Can you work these out from the model? Positions are in its coordinate system, mm. Face numbers are marked on the shaded views. A direction names the side the tool comes from. Round coordinates to 2 decimals unless told otherwise and drop trailing zeros. Loops run counter-clockwise (first coordinate to the right, second up) from the corner with the lowest first, then second, coordinate; pieces in that order, holes last.
(1) I want a section at A-A on x = 10.75. Write out the boundary of the cut face in (y, z), plus the area to 3 significant figures.
(2) I want a section at B-B on y = -11. Write out the boundary of the cut face in (x, z), plus the area to 3 significant figures.
(3) Will these pins go through, and if not, where does the flat tip stop? pin 1 Ø0.5 at (x, z) = (4, -18.5) entering from -Y; pin 2 Ø5.5 at (y, z) = (-0.5, -9) entering from -X.
(4) Which directions (+Z, -Z, +X, -X, +Y, -Y) give clear straight access to the entire face, cutting with the end or side of a thin tool? Please do the marked faces 5, 6, 7 and 8.
(5) Thinking about a two-plate mould opening in X: for the marked faces 1, 2, 3 and 4, which applies, released by +X, released by -X, zero draft, split by the parting line, or undercut?
(6) I want a section at C-C on y = -8.25. Write out the boundary of the cut face in (x, z) (3 decimals).
(7) If I drill on line 1 along Z through (x, y) = (19, -5.5); line 2 along Z through (x, y) = (24.5, 3); line 3 along Y through (x, z) = (25.25, -12) (3 decimals), over which ranges is the centre line in solid material (lowest first)?
from build123d import *

# Parameters (mm, degrees)
BLANKSKE_W           = 27
BLANKSKE_H           = 13.325
BLANK_DEPTH          = 29
TOOTHCUTSIM_DEPTH    = 42.803775248
TEETHCUTS_COUNT      = 8
TEETHCUTS_PITCH      = 3.926990813
CUT_EXTRUDE1_DEPTH   = 6.75
SKETCH3_R            = 5.25
CUT_EXTRUDE2_DEPTH   = 10.25
SKETCH4_R            = 4.5
CUT_EXTRUDE3_DEPTH   = 37.16013862
SKETCH5_R            = 2.5
CUT_EXTRUDE4_DEPTH   = 3.175
SKETCH6_R            = 1.75
CUT_EXTRUDE5_DEPTH   = 40.826953813
MIRROR1_COPY_1_DEPTH = 42.803775248
MIRROR1_COPY_2_DEPTH = 42.803775248
MIRROR1_COPY_3_DEPTH = 42.803775248
MIRROR1_COPY_4_DEPTH = 42.803775248
MIRROR1_COPY_5_DEPTH = 42.803775248
MIRROR1_COPY_6_DEPTH = 42.803775248
MIRROR1_COPY_7_DEPTH = 42.803775248
SKETCH9_W            = 18.526
SKETCH9_H            = 18.526
CUT_EXTRUDE6_DEPTH   = 3.175


with BuildPart() as part:
    # BlankSke → Blank (new body)
    with BuildSketch(Plane.XY):
        with Locations((13.5, 6.6625)):
            Rectangle(BLANKSKE_W, BLANKSKE_H)
    blank = extrude(amount=-BLANK_DEPTH)

    # TooCutSkeSim → ToothCutSim (cut, through all)
    with BuildSketch(Plane.XY):
        Polygon((0.548044212, 10.5125), (-0.548044212, 10.5125), (-1.58095534, 13.3504), (1.58095534, 13.3504), align=None)
    toothcutsim = extrude(amount=-TOOTHCUTSIM_DEPTH, mode=Mode.SUBTRACT)

    # TeethCuts: ToothCutSim ×8
    with Locations(*[(i * TEETHCUTS_PITCH, 0, 0) for i in range(1, TEETHCUTS_COUNT)]):
        add(toothcutsim, mode=Mode.SUBTRACT)

    # Sketch2 → Cut-Extrude1 (cut)
    with BuildSketch(Plane.ZY):
        with BuildLine():
            Line((-7.445049185, 8.763), (-21.554950815, 8.763))
            ThreePointArc((-21.554950815, 8.763), (-24.647184256, 4.857689952), (-25.75, 0))
            Line((-25.75, 0), (-3.25, 0))
            ThreePointArc((-3.25, 0), (-4.352815744, 4.857689952), (-7.445049185, 8.763))
        make_face()
    cut_extrude1 = extrude(amount=-CUT_EXTRUDE1_DEPTH, mode=Mode.SUBTRACT)

    # Sketch3 → Cut-Extrude2 (cut)
    with BuildSketch(Plane.ZY.offset(-6.75)):
        with Locations((-14.5, 0)):
            Circle(SKETCH3_R)
    cut_extrude2 = extrude(amount=-CUT_EXTRUDE2_DEPTH, mode=Mode.SUBTRACT)

    # Sketch4 → Cut-Extrude3 (cut, symmetric)
    with BuildSketch(Plane.ZY.offset(-17)):
        with Locations((-14.5, 0)):
            Circle(SKETCH4_R)
    cut_extrude3 = extrude(amount=CUT_EXTRUDE3_DEPTH, both=True, mode=Mode.SUBTRACT)

    # Sketch5 → Cut-Extrude4 (cut)
    with BuildSketch(Plane(origin=(27, 0, 0), x_dir=(0, 0, -1), z_dir=(1, 0, 0))):
        with Locations((8.932241205, 5.567758795)):
            Circle(SKETCH5_R)
        with Locations((20.067758795, 5.567758795)):
            Circle(SKETCH5_R)
    cut_extrude4 = extrude(amount=-CUT_EXTRUDE4_DEPTH, mode=Mode.SUBTRACT)

    # Sketch6 → Cut-Extrude5 (cut, through all)
    with BuildSketch(Plane(origin=(23.825, 0, 0), x_dir=(0, 0, -1), z_dir=(1, 0, 0))):
        with Locations((20.067758795, 5.567758795)):
            Circle(SKETCH6_R)
        with Locations((8.932241205, 5.567758795)):
            Circle(SKETCH6_R)
    cut_extrude5 = extrude(amount=-CUT_EXTRUDE5_DEPTH, mode=Mode.SUBTRACT)

    # Mirror1: Blank, ToothCutSim, Cut-Extrude1, Cut-Extrude2, Cut-Extrude3, Cut-Extrude4, Cut-Extrude5 across plane
    add(blank.mirror(Plane(origin=(0, 0, -29), x_dir=(0, 0, 1), z_dir=(0, -1, 0))))
    add(toothcutsim.mirror(Plane(origin=(0, 0, -29), x_dir=(0, 0, 1), z_dir=(0, -1, 0))), mode=Mode.SUBTRACT)
    add(cut_extrude1.mirror(Plane(origin=(0, 0, -29), x_dir=(0, 0, 1), z_dir=(0, -1, 0))), mode=Mode.SUBTRACT)
    add(cut_extrude2.mirror(Plane(origin=(0, 0, -29), x_dir=(0, 0, 1), z_dir=(0, -1, 0))), mode=Mode.SUBTRACT)
    add(cut_extrude3.mirror(Plane(origin=(0, 0, -29), x_dir=(0, 0, 1), z_dir=(0, -1, 0))), mode=Mode.SUBTRACT)
    add(cut_extrude4.mirror(Plane(origin=(0, 0, -29), x_dir=(0, 0, 1), z_dir=(0, -1, 0))), mode=Mode.SUBTRACT)
    add(cut_extrude5.mirror(Plane(origin=(0, 0, -29), x_dir=(0, 0, 1), z_dir=(0, -1, 0))), mode=Mode.SUBTRACT)

    # Mirror1 copy 1 sketch → Mirror1 copy 1 (cut, through all)
    with BuildSketch(Plane(origin=(3.926990813, 0, 0), x_dir=(1, 0, 0), z_dir=(0, 0, 1))):
        Polygon((0.548044212, -10.5125), (-0.548044212, -10.5125), (-1.58095534, -13.3504), (1.58095534, -13.3504), align=None)
    extrude(amount=-MIRROR1_COPY_1_DEPTH, mode=Mode.SUBTRACT)

    # Mirror1 copy 2 sketch → Mirror1 copy 2 (cut, through all)
    with BuildSketch(Plane(origin=(7.853981625, 0, 0), x_dir=(1, 0, 0), z_dir=(0, 0, 1))):
        Polygon((0.548044212, -10.5125), (-0.548044212, -10.5125), (-1.58095534, -13.3504), (1.58095534, -13.3504), align=None)
    extrude(amount=-MIRROR1_COPY_2_DEPTH, mode=Mode.SUBTRACT)

    # Mirror1 copy 3 sketch → Mirror1 copy 3 (cut, through all)
    with BuildSketch(Plane(origin=(11.780972438, 0, 0), x_dir=(1, 0, 0), z_dir=(0, 0, 1))):
        Polygon((0.548044212, -10.5125), (-0.548044212, -10.5125), (-1.58095534, -13.3504), (1.58095534, -13.3504), align=None)
    extrude(amount=-MIRROR1_COPY_3_DEPTH, mode=Mode.SUBTRACT)

    # Mirror1 copy 4 sketch → Mirror1 copy 4 (cut, through all)
    with BuildSketch(Plane(origin=(15.70796325, 0, 0), x_dir=(1, 0, 0), z_dir=(0, 0, 1))):
        Polygon((0.548044212, -10.5125), (-0.548044212, -10.5125), (-1.58095534, -13.3504), (1.58095534, -13.3504), align=None)
    extrude(amount=-MIRROR1_COPY_4_DEPTH, mode=Mode.SUBTRACT)

    # Mirror1 copy 5 sketch → Mirror1 copy 5 (cut, through all)
    with BuildSketch(Plane(origin=(19.634954063, 0, 0), x_dir=(1, 0, 0), z_dir=(0, 0, 1))):
        Polygon((0.548044212, -10.5125), (-0.548044212, -10.5125), (-1.58095534, -13.3504), (1.58095534, -13.3504), align=None)
    extrude(amount=-MIRROR1_COPY_5_DEPTH, mode=Mode.SUBTRACT)

    # Mirror1 copy 6 sketch → Mirror1 copy 6 (cut, through all)
    with BuildSketch(Plane(origin=(23.561944875, 0, 0), x_dir=(1, 0, 0), z_dir=(0, 0, 1))):
        Polygon((0.548044212, -10.5125), (-0.548044212, -10.5125), (-1.58095534, -13.3504), (1.58095534, -13.3504), align=None)
    extrude(amount=-MIRROR1_COPY_6_DEPTH, mode=Mode.SUBTRACT)

    # Mirror1 copy 7 sketch → Mirror1 copy 7 (cut, through all)
    with BuildSketch(Plane(origin=(27.488935688, 0, 0), x_dir=(1, 0, 0), z_dir=(0, 0, 1))):
        Polygon((0.548044212, -10.5125), (-0.548044212, -10.5125), (-1.58095534, -13.3504), (1.58095534, -13.3504), align=None)
    extrude(amount=-MIRROR1_COPY_7_DEPTH, mode=Mode.SUBTRACT)

    # Sketch9 → Cut-Extrude6 (cut)
    with BuildSketch(Plane(origin=(27, 0, 0), x_dir=(0, 0, -1), z_dir=(1, 0, 0))):
        with Locations((14.5, 0)):
            Rectangle(SKETCH9_W, SKETCH9_H)
    extrude(amount=-CUT_EXTRUDE6_DEPTH, mode=Mode.SUBTRACT)


solid = part.part
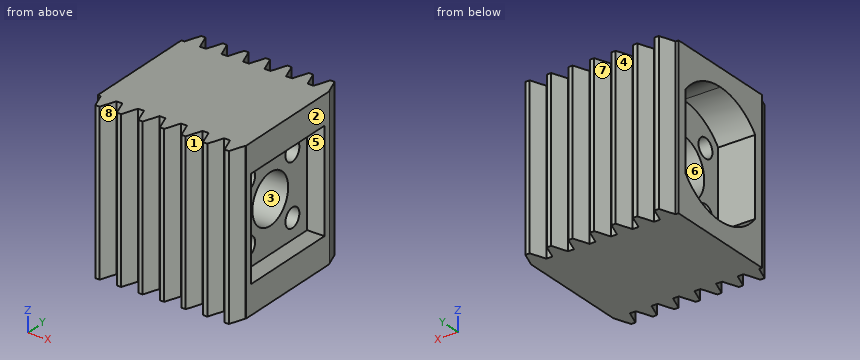
Filled sheet:
1. outline: (-11.84, -29) - (11.84, -29) - (11.84, 0) - (-11.84, 0) - close; hole circle Ø3.5 at (-5.57, -20.07); hole circle Ø3.5 at (-5.57, -8.93); hole circle Ø10.5 at (0, -14.5); hole circle Ø3.5 at (5.57, -20.07); hole circle Ø3.5 at (5.57, -8.93)
1. area: 562 mm2
2. outline: (0.73, -29) - (3.2, -29) - (3.2, 0) - (0.73, 0) - close; (4.65, -29) - (7.13, -29) - (7.13, 0) - (4.65, 0) - close; (8.58, -29) - (11.06, -29) - (11.06, 0) - (8.58, 0) - close; (12.51, -29) - (14.98, -29) - (14.98, 0) - (12.51, 0) - close; (16.43, -29) - (18.91, -29) - (18.91, 0) - (16.43, 0) - close; (20.36, -29) - (22.84, -29) - (22.84, 0) - (20.36, 0) - close; (24.29, -29) - (26.76, -29) - (26.76, 0) - (24.29, 0) - close
2. area: 503 mm2
3. pin 1: stops at y = -10.51
3. pin 2: stops at x = 6.75
4. face 5: +X
4. face 6: -X
4. face 7: +Z, -Z, +Y
4. face 8: +Z, -Z, -Y
5. face 1: undercut
5. face 2: released by +X
5. face 3: zero draft
5. face 4: undercut
6. outline: (0, -29) - (27, -29) - (27, -23.763) - (23.825, -23.763) - (23.825, -5.237) - (27, -5.237) - (27, 0) - (0, 0) - (0, -6.851) - (6.75, -6.851) - (6.75, -22.149) - (0, -22.149) - close
7. line 1: z = -29 to -21.82, -18.32 to -10.68, -7.18 to 0
7. line 2: z = -29 to -23.76, -5.24 to 0
7. line 3: y = -13.325 to -9.263, 9.263 to 13.325
